Design review of the part built by this model. Coordinates are the model's own, in mm. A direction names the side the tool comes from. Coordinates: 2 decimals unless noted, no trailing zeros. Write each loop counter-clockwise with the first axis right and the second up, starting at its lowest first coordinate (ties: lowest second). Pieces come first, ordered by that corner, then holes.
Q1. Insertion check: pin 1 (8.5 mm diameter, centred on x = -14.74, y = -18.66, fed in from +Z); pin 2 (4 mm diameter, centred on x = 8.79, y = 22.1, fed in from +Z); pin 3 (2.5 mm diameter, centred on x = 2, z = 10.5, fed in from +Y); pin 4 (1 mm diameter, centred on y = -31.5, z = 2, fed in from +X). Each pin has a flat end and moves straight along its axis. Give the tip position at first contact, or say it passes through.
Q2. Take a section at B-B (y = 36.5). Give the boundary of the cut face in (x, z), and give its area (3 significant figures).
Q3. Machinability: for faces 4 (the flat face through (0, -7, 8.636)), 5 (the flat face through (-12, 12, 11.938)), which of the approach directions +Z, -Z, +X, -X, +Y, -Y give a long, thin tool a straight path to every point of the face, cutting with its end or side? Answer none if there is none.
Q4. For probe 1 along Y at (x, z) = (4, 11.75); probe 2 along X at (y, z) = (-29.5, 9); probe 3 along Z at (x, y) = (-5, 6.5), list the stretches that pass through material, from the lowest coordinate up.
Q5. Take a section at D-D (x = -41). Give the boundary of the cut face in (y, z).
Q6. Mouldability with a two-part tool opening along Y and no side actions: class faces 1 (the cylindrical face through (11.65, -19.38, 9.59)), 2 (the flat face through (11, 1, 0)), 3 (the flat face through (0, 41.402, 10)) as pulls with the +Y half, pulls with the -Y half, needs draft (parallel to the pull), parting line crosses it, or undercut.
Q7. Take a section at C-C (z = 3.5). Give the boundary of the cut face in (x, y).
Q8. Take a section at A-A (x = 0). Give the boundary of the cut face in (y, z), and give its area (3 significant figures).
```python
from build123d import *

# Parameters (mm, degrees)
SKETCH1_R                = 50.8
BASEPLATE_DEPTH          = 11.938
SKETCH3_R                = 16.03375
MAGNET_INSET_DEPTH       = 3.302
SKETCH4_W                = 17.575320152
SKETCH4_H                = 19.304
DOWEL_SLOT_DEPTH         = 4.7625
SKETCH6_R                = 3.175
DOWEL_SLOT_RELIEFS_DEPTH = 4.7625
DOWEL_SLOT_PATTERN_COUNT = 3
SKETCH7_R                = 6.35
CENTRAL_HOLE_DEPTH       = 73.82716419


with BuildPart() as part:
    # Sketch1 → baseplate (new body)
    with BuildSketch(Plane.XY):
        Circle(SKETCH1_R)
    extrude(amount=BASEPLATE_DEPTH)

    # Sketch3 → magnet_inset (cut)
    with BuildSketch(Plane.XY.offset(11.938)):
        Circle(SKETCH3_R)
    extrude(amount=-MAGNET_INSET_DEPTH, mode=Mode.SUBTRACT)

    # Sketch4 → dowel_slot (cut)
    with BuildSketch(Plane.XY.offset(11.938)):
        with Locations((0, 31.75)):
            Rectangle(SKETCH4_W, SKETCH4_H)
    dowel_slot = extrude(amount=-DOWEL_SLOT_DEPTH, mode=Mode.SUBTRACT)

    # Sketch6 → dowel_slot_reliefs (cut)
    with BuildSketch(Plane.XY.offset(11.938)):
        with Locations((-8.787660076, 41.402)):
            Circle(SKETCH6_R)
        with Locations((8.787660076, 41.402)):
            Circle(SKETCH6_R)
        with Locations((8.787660076, 22.098)):
            Circle(SKETCH6_R)
        with Locations((-8.787660076, 22.098)):
            Circle(SKETCH6_R)
    dowel_slot_reliefs = extrude(amount=-DOWEL_SLOT_RELIEFS_DEPTH, mode=Mode.SUBTRACT)

    # dowel_slot_pattern: dowel_slot, dowel_slot_reliefs ×3 about axis
    dowel_slot_pattern_axis = Axis((0, 0, 0), (0, 0, 1))
    add([dowel_slot.rotate(dowel_slot_pattern_axis, i * 360 / DOWEL_SLOT_PATTERN_COUNT) for i in range(1, DOWEL_SLOT_PATTERN_COUNT)], mode=Mode.SUBTRACT)
    add([dowel_slot_reliefs.rotate(dowel_slot_pattern_axis, i * 360 / DOWEL_SLOT_PATTERN_COUNT) for i in range(1, DOWEL_SLOT_PATTERN_COUNT)], mode=Mode.SUBTRACT)

    # Sketch7 → central_hole (cut, through all)
    with BuildSketch(Plane.XY.offset(11.938)):
        Circle(SKETCH7_R)
    extrude(amount=-CENTRAL_HOLE_DEPTH, mode=Mode.SUBTRACT)


solid = part.part
```
Response:
1. pin 1: stops at z = 11.94
1. pin 2: stops at z = 7.18
1. pin 3: stops at y = 50.79
1. pin 4: stops at x = 40.24
2. outline: (-35.33, 0) - (35.33, 0) - (35.33, 11.94) - (8.79, 11.94) - (8.79, 7.18) - (-8.79, 7.18) - (-8.79, 11.94) - (-35.33, 11.94) - close
2. area: 760 mm2
3. face 4: +Z
3. face 5: +Z, +X, -X, +Y, -Y
4. probe 1: y = -50.64 to -15.53, 15.53 to 22.1, 41.4 to 50.64
4. probe 2: x = -41.36 to -34.41, -28.52 to 28.52, 34.41 to 41.36
4. probe 3: z = 0 to 8.64
5. outline: (-29.99, 0) - (29.99, 0) - (29.99, 11.94) - (-10.01, 11.94) - (-10.01, 7.18) - (-16.18, 7.18) - (-16.18, 11.94) - (-29.99, 11.94) - close
6. face 1: undercut
6. face 2: needs draft
6. face 3: undercut
7. outline: circle Ø101.6 at (0, 0); hole circle Ø12.7 at (0, 0)
8. outline: (-50.8, 0) - (-6.35, 0) - (-6.35, 8.64) - (-16.03, 8.64) - (-16.03, 11.94) - (-50.8, 11.94) - close; (6.35, 0) - (50.8, 0) - (50.8, 11.94) - (41.4, 11.94) - (41.4, 7.18) - (22.1, 7.18) - (22.1, 11.94) - (16.03, 11.94) - (16.03, 8.64) - (6.35, 8.64) - close
8. area: 905 mm2
